Source: CAD feature listing. Evaluate the final solid. Frame: model axes, mm. Face numbers are marked on the shaded views. A direction names the side the tool comes from. Coordinates: 2 decimals unless noted, no trailing zeros. Loops run counter-clockwise (first coordinate to the right, second up) from the corner with the lowest first, then second, coordinate; pieces in that order, holes last. Notation, with made-up numbers: (-39, -28.75) -> (-30, -28.75) arc R37 ccw to (-30, 10.25) -> close; hole circle Ø4 at (-6.5, -6). An arc over 180 degrees is marked (long way). One line per question, with ' | ' between items. Start each with the question number.
```python
from build123d import *

# Parameters (mm, degrees)
F0_R     = 4.2164
F1_DEPTH = 3.048
F3_W     = 25.4
F3_H     = 44.704
F5_DEPTH = 3.048
F4_W     = 50.8
F4_H     = 25.4
F6_DEPTH = 3.048
F2_W     = 25.4
F2_H     = 44.704
F7_DEPTH = 3.048
F8_R     = 2.54


with BuildPart() as f1:
    # F0 (on Front) → F1 (new body)
    with BuildSketch(Plane.XZ):
        Polygon((29.872065, 25.170984), (-33.119935, 25.170984), (-33.119935, -19.533016), (-27.023935, -19.533016), (-27.023935, -25.878732), (23.776065, -25.878732), (23.776065, -19.533016), (29.872065, -19.533016), align=None)
        with Locations((-14.323935, 15.010984)):
            Circle(F0_R, mode=Mode.SUBTRACT)
        with Locations((11.076065, 15.010984)):
            Circle(F0_R, mode=Mode.SUBTRACT)
    extrude(amount=F1_DEPTH)

    # F3 (on face) → F5 (join)
    with BuildSketch(Plane(origin=(-33.119935, 0, 0), x_dir=(0, -1, 0), z_dir=(-1, 0, 0))):
        with Locations((-12.7, 2.818984)):
            Rectangle(F3_W, F3_H)
        with BuildLine():
            Line((-20.32, -11.913016), (-20.32, 17.550984))
            ThreePointArc((-20.32, 17.550984), (-17.78, 20.090984), (-15.24, 17.550984))
            Line((-15.24, 17.550984), (-15.24, -11.913016))
            ThreePointArc((-15.24, -11.913016), (-17.78, -14.453016), (-20.32, -11.913016))
        make_face(mode=Mode.SUBTRACT)
    extrude(amount=-F5_DEPTH)

    # F4 (on face) → F6 (join)
    with BuildSketch(Plane(origin=(0, 0, -25.878732), x_dir=(1, 0, 0), z_dir=(0, 0, -1))):
        with Locations((-1.623935, -12.7)):
            Rectangle(F4_W, F4_H)
        with BuildLine():
            ThreePointArc((-19.403935, -21.59), (-21.943935, -19.05), (-19.403935, -16.51))
            Line((-19.403935, -16.51), (16.156065, -16.51))
            ThreePointArc((16.156065, -16.51), (18.696065, -19.05), (16.156065, -21.59))
            Line((16.156065, -21.59), (-19.403935, -21.59))
        make_face(mode=Mode.SUBTRACT)
    extrude(amount=-F6_DEPTH)

    # F2 (on face) → F7 (join)
    with BuildSketch(Plane.YZ.offset(29.872065)):
        with Locations((12.7, 2.818984)):
            Rectangle(F2_W, F2_H)
    extrude(amount=-F7_DEPTH)

    # F8
    f8_edges = [f1.edges().sort_by_distance(p)[0] for p in [
        (-33.119935, -3.048, 2.818984),
        (-30.071935, 0, 2.818984),
        (29.872065, -3.048, 2.818984),
        (26.824065, 0, 2.818984),
        (-1.623935, 0, -22.830732),
        (-1.623935, -3.048, -25.878732),
    ]]
    fillet(f8_edges, radius=F8_R)


solid = f1.part
```
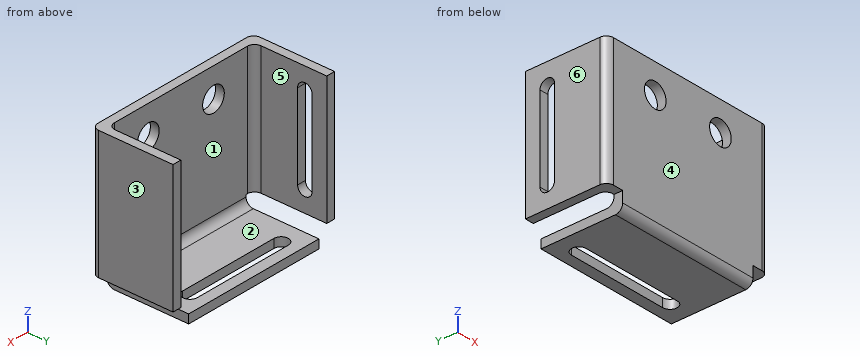
(1) Cut plane B-B, the plane y = 7.5. Return the cut outline in (x, z).
(2) Draft query along X for the marked faces 4, 5 and 6. Return one class per face: pulls with the +X half, pulls with the -X half, needs draft (parallel to the pull), parting line crosses it, or undercut.
(3) Cut plane C-C, the plane x = -0.5. Return the cut outline in (y, z).
(4) Access query for the marked faces 1, 2 and 3. Directions: +Z, -Z, +X, -X, +Y, -Y. A direction counts if a zero-diameter tool reaches every point of the face in a straight line with its end or side. Return the directions, or none.
(5) Cut plane A-A, the plane z = -5.5. Return the cut outline in (x, y).
(6) Contact query for flat-ended pins moving along their axis: pin 1 Ø11.5 at (x, y) = (-2.5, 10) entering from +Z; pin 2 Ø22.5 at (x, z) = (8.5, -6.5) entering from +Y; pin 3 Ø3 at (y, z) = (11.5, -22.5) entering from +X. Output: stop coordinate, or through.
(7) Ray query, L1, parallel to X at y = 14, z = -15; L2, parallel to Z at x = -9, y = 13.25; L3, parallel to Y at x = 12.5, z = -20. Return the intervals inside material, ascending.
(8) Cut plane D-D, the plane y = 19.05. Return the cut outline in (x, z).
Here are the results:
1) outline: (-33.12, -19.53) -> (-30.07, -19.53) -> (-30.07, 25.17) -> (-33.12, 25.17) -> close; (-27.02, -25.88) -> (23.78, -25.88) -> (23.78, -22.83) -> (-27.02, -22.83) -> close; (26.82, -19.53) -> (29.87, -19.53) -> (29.87, 25.17) -> (26.82, 25.17) -> close
2) face 4: needs draft | face 5: undercut | face 6: pulls with the -X half
3) outline: (-3.05, -23.34) arc R2.54 ccw to (-0.51, -25.88) -> (16.51, -25.88) -> (16.51, -22.83) -> (2.54, -22.83) arc R2.54 cw to (0, -20.29) -> (0, 25.17) -> (-3.05, 25.17) -> close; (21.59, -25.88) -> (25.4, -25.88) -> (25.4, -22.83) -> (21.59, -22.83) -> close
4) face 1: +Z, +Y | face 2: +Z, +X, -X, +Y | face 3: +Z, -Z, +X, +Y, -Y
5) outline: (-33.12, -0.51) arc R2.54 ccw to (-30.58, -3.05) -> (27.33, -3.05) arc R2.54 ccw to (29.87, -0.51) -> (29.87, 25.4) -> (26.82, 25.4) -> (26.82, 2.54) arc R2.54 cw to (24.28, 0) -> (-27.53, 0) arc R2.54 cw to (-30.07, 2.54) -> (-30.07, 15.24) -> (-33.12, 15.24) -> close; (-33.12, 20.32) -> (-30.07, 20.32) -> (-30.07, 25.4) -> (-33.12, 25.4) -> close
6) pin 1: stops at z = -22.83 | pin 2: stops at y = 0 | pin 3: stops at x = 23.78
7) L1: x = -33.12 to -30.07, 26.82 to 29.87 | L2: z = -25.88 to -22.83 | L3: y = -3.05 to 0
8) outline: (-33.12, -19.53) -> (-30.07, -19.53) -> (-30.07, -14.11) -> (-33.12, -14.11) -> close; (-33.12, 19.75) -> (-30.07, 19.75) -> (-30.07, 25.17) -> (-33.12, 25.17) -> close; (-27.02, -25.88) -> (-21.94, -25.88) -> (-21.94, -22.83) -> (-27.02, -22.83) -> close; (18.7, -25.88) -> (23.78, -25.88) -> (23.78, -22.83) -> (18.7, -22.83) -> close; (26.82, -19.53) -> (29.87, -19.53) -> (29.87, 25.17) -> (26.82, 25.17) -> close
